The model under review builds one solid part; all positions refer to its coordinate system, in mm. Round coordinates to 2 decimals unless told otherwise and drop trailing zeros. Write each loop counter-clockwise with the first axis right and the second up, starting at its lowest first coordinate (ties: lowest second). Pieces come first, ordered by that corner, then holes. Notation, with made-up numbers: (9.5, 40.5) - (26.5, 40.5) arc R17 ccw to (26.5, 57.5) - close; hole circle Ø3 at (-37.5, 25.5). An arc over 180 degrees is marked (long way). Write each question's results on one line, items separated by ' | '.
```python
from build123d import *

# Parameters (mm, degrees)
SKETCH2_R           = 4.8768
SKETCH2_R_2         = 3.96875
BOSS_EXTRUDE1_DEPTH = 9.525
BOSS_EXTRUDE2_START = 9.525
SKETCH3_R           = 6.35
SKETCH3_R_2         = 3.96875
BOSS_EXTRUDE2_DEPTH = 9.525
DRAFT1_ANGLE        = -3


with BuildPart() as part:
    # Sketch2 → Boss-Extrude1 (new body)
    with BuildSketch(Plane.XY):
        with Locations(Location((0, 0, 0), (0, 0, 180))):
            Circle(SKETCH2_R)
        with Locations(Location((0, 0, 0), (0, 0, 180))):
            Circle(SKETCH2_R_2, mode=Mode.SUBTRACT)
    extrude(amount=BOSS_EXTRUDE1_DEPTH)

    # Sketch3 → Boss-Extrude2 (add)
    with BuildSketch(Plane(origin=(0, 0, 0), x_dir=(-1, 0, 0), z_dir=(0, 0, -1)).offset(BOSS_EXTRUDE2_START)):
        with Locations(Location((0, 0, 0), (0, 0, 180))):
            Circle(SKETCH3_R)
        Circle(SKETCH3_R_2, mode=Mode.SUBTRACT)
    extrude(amount=-BOSS_EXTRUDE2_DEPTH)

    # Draft1
    draft1_faces = [part.faces().sort_by_distance(p)[0] for p in [
        (-6.35, 0, -4.7625),
    ]]
    draft(draft1_faces, Plane.XY, DRAFT1_ANGLE)


solid = part.part
```
Q1. We need section A-A (x = 0). State the section outline as (y, z) points (3 decimals), plus the area to 3 significant figures.
Evaluation:
outline: (-6.35, 0) - (-5.851, -9.525) - (-3.969, -9.525) - (-3.969, 9.525) - (-4.877, 9.525) - (-4.877, 0) - close; (3.969, -9.525) - (5.851, -9.525) - (6.35, 0) - (4.877, 0) - (4.877, 9.525) - (3.969, 9.525) - close | area: 57.9 mm^2
Q2. The part is to be moulded in two halves that separate along Z. For faces 1 (the conical face through (5.815, -1.831, -4.829)), 2 (the flat face through (-1, 5, 0)), 3 (the cylindrical face through (-4.652, -1.465, 4.696)), say which applies: released by +Z, released by -Z, zero draft, split by the parting line, or undercut.
Evaluation:
face 1: released by -Z | face 2: released by +Z | face 3: zero draft
Q3. We need section C-C (z = 7.25). State the section outline as (x, y) points, plus the area to 3 significant figures.
Evaluation:
outline: circle Ø9.75 at (0, 0); hole circle Ø7.94 at (0, 0) | area: 25.2 mm^2
Q4. For probe 1 along Y at (x, z) = (0, 7); probe 2 along Z at (x, y) = (4.75, 1.25) (3 decimals); probe 3 along Y at (x, z) = (-1.5, 3), list the stretches that pass through material, from the lowest coordinate up.
Evaluation:
probe 1: y = -4.88 to -3.97, 3.97 to 4.88 | probe 2: z = -9.525 to 0 | probe 3: y = -4.64 to -3.67, 3.67 to 4.64
Q5. We need section D-D (z = -0.25). State the section outline as (x, y) points.
Evaluation:
outline: circle Ø12.67 at (0, 0); hole circle Ø7.94 at (0, 0)
Q6. Insertion check: P1, Ø5, axis at x = -1.5, z = -7, coming from the +Y side; P2, Ø5, axis at x = 4.5, y = 4.5, coming from the -Z side (3 decimals); P3, Ø5, axis at x = 1, z = -5.5, coming from the -Y side; P4, Ø2, axis at x = -5, z = 4.5, coming from the +Y side. Each pin has a flat end and moves straight along its axis. Give the tip position at first contact, or say it passes through.
Evaluation:
P1: stops at y = 6.09 | P2: stops at z = -9.525 | P3: stops at y = -6.18 | P4: stops at y = 2.79
